CAD build for the part. Positions are in the model's coordinates, mm. Face numbers are marked on the shaded views. A direction names the side the tool comes from. Round coordinates to 2 decimals unless told otherwise and drop trailing zeros. Order: outer loops, then holes, each group sorted by start corner. A loop starts at its lowest first (then second) coordinate and runs counter-clockwise, first axis right, second up. Notation, with made-up numbers: M -33.5,17 L 13.5,17 A28 ccw 13.5,37 Z; hole C 78.5,-39.5 d9. An arc over 180 degrees is marked long. Answer as a JSON object with one key per item and string values.
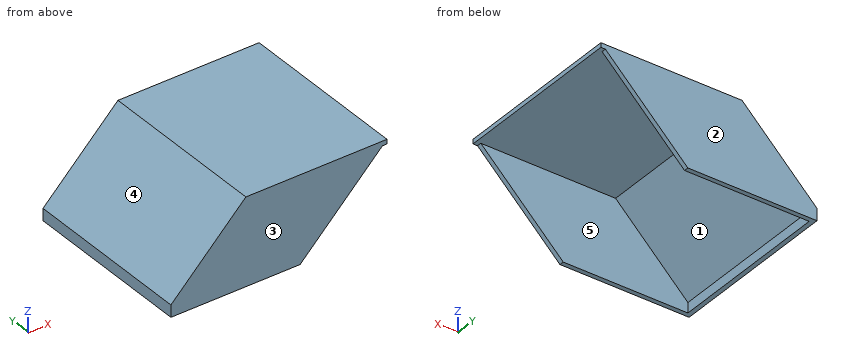
Autodesk Inventor part; units mm, degrees
ref_plane "РабПлоскость1" through (-68.51, -58, -55) normal (0, 0, 1) x (1, 0, 0)
ref_plane "YZ Plane" through (0, 0, 0) normal (1, 0, 0) x (0, 1, 0)
ref_plane "XZ Plane" through (0, 0, 0) normal (0, 1, 0) x (-1, 0, 0)
sketch "Эскиз1" plane through (0, 0, 0) normal (0, 0, 1) x (1, 0, 0)
  line L0 (-77.0756, -58) -> (-77.0756, 58)
  line L1 (-77.0756, 58) -> (67.0756, 58)
  line L2 (67.0756, 58) -> (67.0756, -58)
  line L3 (67.0756, -58) -> (-77.0756, -58)
  line L4 (-77.0756, -58) -> (-77.0756, 58)
  line L5 (9.0756, -58) -> (-77.0756, -58)
  line L6 (-77.0756, 58) -> (9.0756, 58)
  point P0 (0, 0)
extrude "Выдавливание1" add sketch "Эскиз1" along normal blind 3
sketch "Эскиз2" plane through (0, 0, 0) normal (0, 0, -1) x (-1, 0, 0)
  line L0 (-64.0756, 55) -> (74.0756, 55)
  line L1 (74.0756, 55) -> (74.0756, -55)
  line L2 (74.0756, -55) -> (-64.0756, -55)
  line L3 (-64.0756, -55) -> (-64.0756, 55)
  line L4 (77.0756, -58) -> (77.0756, 58)
  line L5 (77.0756, 58) -> (-67.0756, 58)
  line L6 (-67.0756, 58) -> (-67.0756, -58)
  line L7 (-67.0756, -58) -> (77.0756, -58)
  line L8 (-67.0756, -58) -> (-67.0756, 58)
  line L9 (-67.0756, 58) -> (77.0756, 58)
  line L10 (77.0756, 58) -> (77.0756, -58)
  line L11 (77.0756, -58) -> (-67.0756, -58)
  line L12 (-9.0756, 55) -> (74.0756, 55)
  line L13 (74.0756, 55) -> (74.0756, -55)
  line L14 (74.0756, -55) -> (-9.0756, -55)
  point P0 (0, 0)
  point P1 (68.51, 55)
  point P2 (68.51, -55)
ref_plane "РабПлоскость1" through (-68.51, -58, -55) normal (0, 0, 1) x (1, 0, 0)
extrude "Выдавливание2" add sketch "Эскиз2" along normal up to surface (55 mm away)
chamfer "Фаска1" distance 50 angle 45 1 edges at (-77.0756, 0, 3)
sketch "Эскиз4" plane through (-27.7928, -58, 2.2828) normal (-0.7071068, 0, 0.7071068) x (0.7071068, 0, 0.7071068)
  line L0 (-3.2284, 3) -> (-65.4538, 3)
  line L1 (-65.4538, 3) -> (-65.4538, 113)
  line L2 (-65.4538, 113) -> (-3.2284, 113)
  line L3 (-3.2284, 113) -> (-3.2284, 3)
  line L4 (-69.6964, 0) -> (1.0143, 0)
  line L5 (1.0143, 0) -> (1.0143, 116)
  line L6 (1.0143, 116) -> (-69.6964, 116)
  line L7 (-69.6964, 116) -> (-69.6964, 0)
  point P0 (18.0383, 58)
extrude "Выдавливание4" add sketch "Эскиз4" against normal blind 3 contours L0 L1 L2 L3 | L7 L6 L5 L4
sketch "Эскиз9" plane through (-28.51, -58, 3) normal (-0.7071068, 0, 0.7071068) x (0.7071068, 0, 0.7071068)
  line L0 (-10, 105.175) -> (-30, 105.175)
  line L1 (-30, 105.175) -> (-30, 91.875)
  line L2 (-30, 91.875) -> (-10, 91.875)
  line L3 (-10, 91.875) -> (-10, 105.175)
  circle A0 centre (-43.2843, 98.525) radius 5.25
  line L4 (-7, 80.55) -> (-33, 80.55)
  line L5 (-33, 80.55) -> (-33, 35.45)
  line L6 (-33, 35.45) -> (-7, 35.45)
  line L7 (-7, 35.45) -> (-7, 80.55)
  line L8 (-33.5, 34.95) -> (-33.5, 81.05)
  line L9 (-33.5, 81.05) -> (-6.5, 81.05)
  line L10 (-6.5, 81.05) -> (-6.5, 34.95)
  line L11 (-6.5, 34.95) -> (-33.5, 34.95)
  line L12 (-6.5, 70.5) -> (-33.5, 70.5)
  line L13 (-33.5, 70.5) -> (-33.5, 45.5)
  line L14 (-33.5, 45.5) -> (-6.5, 45.5)
  line L15 (-6.5, 45.5) -> (-6.5, 70.5)
  line L16 (-6.5, 70.5) -> (-6, 70.5)
  line L17 (-6, 70.5) -> (-6, 45.5)
  line L18 (-6, 45.5) -> (-6.5, 45.5)
  line L19 (-6.5, 45.5) -> (-6.5, 70.5)
  line L20 (-33.5, 70.5) -> (-34, 70.5)
  line L21 (-34, 70.5) -> (-34, 45.5)
  line L22 (-34, 45.5) -> (-33.5, 45.5)
  line L23 (-33.5, 45.5) -> (-33.5, 70.5)
  line L24 (0, 0) -> (0, 116)
  line L25 (0, 116) -> (0, 0)
  line L26 (0, 0) -> (0, 58)
  line L27 (0, 58) -> (-56.5685, 58)
  line L28 (-56.5685, 116) -> (-56.5685, 0)
  circle A1 centre (-15.7843, 17.475) radius 3.65
  circle A2 centre (-40.7843, 17.475) radius 3.65
  line L29 (-6.5, 34.95) -> (-6.5, 0)
  line L30 (-56.5685, 0) -> (0, 0)
  line L31 (-6.5, 17.475) -> (-56.5685, 17.475)
  line L32 (-56.5685, 17.475) -> (0, 17.475)
  line L33 (-15.7843, 17.475) -> (-40.7843, 17.475)
  circle A3 centre (-45.0343, 73.55) radius 4.15
  line L34 (-56.5685, 81.05) -> (-33.5, 81.05)
  line L35 (-33.5, 81.05) -> (-33.5, 34.95)
  line L36 (-33.5, 34.95) -> (-56.5685, 34.95)
  line L37 (-56.5685, 34.95) -> (-56.5685, 81.05)
  line L38 (-45.0343, 81.05) -> (-45.0343, 34.95)
  circle A4 centre (-45.0343, 73.55) radius 7.5
  line L39 (-6.5, 81.05) -> (-6.5, 116)
  line L40 (-6.5, 98.525) -> (-56.5685, 98.525)
  line L41 (-56.5685, 98.525) -> (0, 98.525)
  line L42 (-30, 98.525) -> (-56.5685, 98.525)
  line L43 (-20, 91.875) -> (-20, 0)
  point P0 (18.0383, 58)
  point P1 (-6.5, 58)
  point P2 (-6.5, 58)
  point P3 (-28.2843, 17.475)
  point P4 (-10, 98.525)
  point P5 (-20, 81.05)
  dimension "d31" = 20
  dimension "d32" = 13.3
  dimension "d33" = 10.5
  dimension "d34" = 26
  dimension "d35" = 45.1
  dimension "d36" = 0.5
  dimension "d37" = 25
  dimension "d38" = 0.5
  dimension "d39" = 0.5
  dimension "d40" = 7.3
  dimension "d41" = 7.3
  dimension "d45" = 25
  dimension "d46" = 8.3
  dimension "d47" = 15
  dimension "d48" = 10
sketch "Эскиз10" plane through (-28.51, -58, 3) normal (-0.7071068, 0, 0.7071068) x (0.7071068, 0, 0.7071068)
  line L0 (-30, 105.175) -> (-30, 91.875)
  line L1 (-10, 105.175) -> (-30, 105.175)
  line L2 (-30, 91.875) -> (-10, 91.875)
  line L3 (-10, 91.875) -> (-10, 105.175)
  circle A0 centre (-43.2843, 98.525) radius 5.25
  circle A1 centre (-45.0343, 73.55) radius 4.15
  circle A2 centre (-40.7843, 17.475) radius 3.65
  circle A3 centre (-15.7843, 17.475) radius 3.65
  line L4 (-6.5, 34.95) -> (-33.5, 34.95)
  line L5 (-33.5, 34.95) -> (-33.5, 81.05)
  line L6 (-34, 70.5) -> (-34, 45.5)
  line L7 (-33.5, 81.05) -> (-6.5, 81.05)
  line L8 (-6.5, 81.05) -> (-6.5, 34.95)
  line L9 (-6.5, 70.5) -> (-6, 70.5)
  line L10 (-6, 70.5) -> (-6, 45.5)
  line L11 (-6, 45.5) -> (-6.5, 45.5)
  line L12 (-33.5, 70.5) -> (-34, 70.5)
  line L13 (-34, 45.5) -> (-33.5, 45.5)
  line L14 (-6.15, 69.35) -> (-6.15, 60.2)
  point P0 (18.0383, 58)
extrude "Выдавливание9" [suppressed]
sketch "Эскиз11" plane through (-25.6715, -58, 0.1615) normal (0.7071068, 0, -0.7071068) x (-0.7071068, 0, -0.7071068)
  line L0 (0.2284, 3) -> (0.2284, 113)
  line L1 (40.7843, 17.475) -> (40.7843, 25.8116)
  line L2 (38.9594, 25.1915) -> (38.9372, 24.9384)
  arc A0 (38.8018, 24.8228) -> (38.9372, 24.9384) centre (38.8107, 24.9495) ccw
  arc A1 (38.8018, 24.8228) -> (37.7667, 24.8228) centre (38.2843, 17.475) ccw
  arc A2 (38.9594, 25.1915) -> (38.8419, 25.3292) centre (38.8329, 25.2026) ccw
  arc A3 (37.6313, 24.9384) -> (37.7667, 24.8228) centre (37.7578, 24.9495) ccw
  line L3 (37.6092, 25.1915) -> (37.6313, 24.9384)
  arc A4 (37.7267, 25.3292) -> (37.6092, 25.1915) centre (37.7357, 25.2026) ccw
  arc A5 (39.3003, 25.2832) -> (37.2683, 25.2832) centre (38.2843, 17.475) ccw
  arc A6 (40.1771, 26.0275) -> (39.4118, 25.1305) centre (40.2357, 25.2026) ccw
  line L4 (39.4118, 25.1305) -> (39.434, 24.8774)
  arc A7 (39.434, 24.8774) -> (40.3159, 24.1245) centre (40.2578, 24.9495) ccw
  arc A8 (41.2526, 24.1245) -> (40.3159, 24.1245) centre (40.7843, 17.475) ccw
  arc A9 (41.2526, 24.1245) -> (42.1346, 24.8774) centre (41.3107, 24.9495) ccw
  line L5 (42.1346, 24.8774) -> (42.1567, 25.1305)
  arc A10 (42.1567, 25.1305) -> (41.3914, 26.0275) centre (41.3329, 25.2026) ccw
  circle A11 centre (40.7843, 17.475) radius 8.574
  arc A12 (-9.3529, 50.5788) -> (-10.2349, 51.3317) centre (-10.1768, 50.5067) ccw
  arc A13 (-11.1715, 51.3317) -> (-10.2349, 51.3317) centre (-10.7032, 57.9812) ccw
  arc A14 (-11.1715, 51.3317) -> (-12.0535, 50.5788) centre (-11.2297, 50.5067) ccw
  arc A15 (-12.0756, 50.3258) -> (-11.3104, 49.4288) centre (-11.2518, 50.2537) ccw
  arc A16 (-10.0961, 49.4288) -> (-9.3308, 50.3258) centre (-10.1546, 50.2537) ccw
  line L6 (-9.3308, 50.3258) -> (-9.3529, 50.5788)
  line L7 (-12.0535, 50.5788) -> (-12.0756, 50.3258)
  circle A17 centre (15.7843, 17.475) radius 8.574
  arc A18 (14.4118, 9.8195) -> (15.1771, 8.9225) centre (15.2357, 9.7474) ccw
  arc A19 (15.3159, 10.8255) -> (14.434, 10.0726) centre (15.2578, 10.0005) ccw
  line L8 (14.434, 10.0726) -> (14.4118, 9.8195)
  arc A20 (15.3159, 10.8255) -> (16.2526, 10.8255) centre (15.7843, 17.475) ccw
  arc A21 (17.1346, 10.0726) -> (16.2526, 10.8255) centre (16.3107, 10.0005) ccw
  arc A22 (16.3914, 8.9225) -> (17.1567, 9.8195) centre (16.3329, 9.7474) ccw
  line L9 (17.1567, 9.8195) -> (17.1346, 10.0726)
  line L10 (0.2284, 113) -> (68.4538, 113)
  line L11 (68.4538, 3) -> (0.2284, 3)
  line L12 (68.4538, 113) -> (68.4538, 3)
  point P0 (-18.0383, 58)
  point P1 (40.1771, 26.0275)
  point P2 (15.1771, 8.9225)
  point P3 (16.3914, 8.9225)
  point P4 (15.1771, 8.9225)
  point P5 (16.3914, 8.9225)
  point P6 (17.1346, 10.0726)
extrude "Выдавливание10" [suppressed]
sketch "Эскиз14" plane through (-65.51, -55, -55) normal (1, 0, 0) x (0, 0, -1)
  line L0 (-55, 0) -> (-55, 110)
  line L1 (-24.0346, 70.55) -> (-16.7574, 70.55)
  line L2 (-16.7574, 110) -> (-16.7574, 0)
  line L3 (-18.0074, 65.55) -> (-15.5074, 65.55)
  line L4 (-15.5074, 65.55) -> (-15.5074, 75.55)
  line L5 (-15.5074, 75.55) -> (-18.0074, 75.55)
  line L6 (-18.0074, 75.55) -> (-18.0074, 65.55)
  line L7 (-18.0074, 65.55) -> (-15.5074, 75.55) construction
  line L8 (-15.5074, 65.55) -> (-18.0074, 75.55) construction
  line L9 (-55, 110) -> (-6.7574, 110)
  line L10 (-6.7574, 0) -> (-55, 0)
  line L11 (-6.7574, 110) -> (-6.7574, 0)
  point P0 (-55, 55)
  dimension "d63" = 2.5
  dimension "d64" = 10
extrude "Выдавливание13" [suppressed]
ref_plane "РабПлоскость2" through (-65.51, 15.55, -39.4926) normal (0, -1, 0) x (1, 0, 0)
sketch "Эскиз15" plane through (-77.0756, 58, -55) normal (0, 1, 0) x (1, 0, 0)
  line L0 (86.1512, 0) -> (141.1512, -55)
  line L1 (144.1512, -55) -> (141.1512, -55)
  line L2 (0, 0) -> (86.1512, 0)
  line L3 (50, -58) -> (0, -8)
  line L4 (144.1512, -58) -> (50, -58)
  line L5 (144.1512, 0) -> (144.1512, -58)
  line L6 (0, 0) -> (144.1512, 0)
  line L7 (0, 0) -> (0, -8)
  point P0 (77.0756, -55)
extrude "Выдавливание14" cut sketch "Эскиз15" against normal up to surface (116 mm away) contours L6 L5 L1 L0
properties part number "LPS_cap"
Item 1: Saw through at B-B on y = 29. List the corners of the cut face in (x, z), and give its area (3 significant figures).
Worked answers:
{"outline": "M -77.08,-55 L -74.08,-55 L -74.08,-48.24 L -25.83,0 L 67.08,0 L 67.08,3 L -27.08,3 L -77.08,-47 Z", "area": "511 mm2"}
Item 2: 3-axis set-ups, long thin cutter, end or side, ignore diameter. For the marked faces 1 and 2: which of +Z, -Z, +X, -X, +Y, -Y reach the whole face in a straight line?
Worked answers:
{"face 1": "-Z, +X", "face 2": "+Z, -Z, +X, -X, +Y"}
Item 3: Drop flat-ended pins along their axis: pin 1 Ø5.5 at (y, z) = (15.5, -52) entering from +X; pin 2 Ø5 at (x, y) = (34.5, -26.5) entering from -Z; pin 3 Ø6 at (y, z) = (-29.5, -37.5) entering from -X. Give the stop position or say it passes through.
Worked answers:
{"pin 1": "stops at x = -74.08", "pin 2": "stops at z = 0", "pin 3": "stops at x = -70.58"}
Item 4: Wall check: line 1 along Y through (x, z) = (-4.5, -16); line 2 along Z through (x, y) = (49.5, 17.5); line 3 along X through (y, z) = (-25, -15.5). Give the ranges that are in metal, low to high. Write a range as [from, to].
Worked answers:
{"line 1": "y = [-58, -55], [55, 58]", "line 2": "z = [0, 3]", "line 3": "x = [-45.58, -41.33]"}
Item 5: Saw through at A-A on x = -10. List the corners of the cut face in (y, z).
Worked answers:
{"outline": "M -58,-55 L -55,-55 L -55,0 L 55,0 L 55,-55 L 58,-55 L 58,3 L -58,3 Z"}
Item 6: Two-plate mould, pull along Y, no slides. Class the marked faces 3, 4 and 5: released by +Y, released by -Y, zero draft, split by the parting line, or undercut.
Worked answers:
{"face 3": "released by -Y", "face 4": "zero draft", "face 5": "undercut"}
